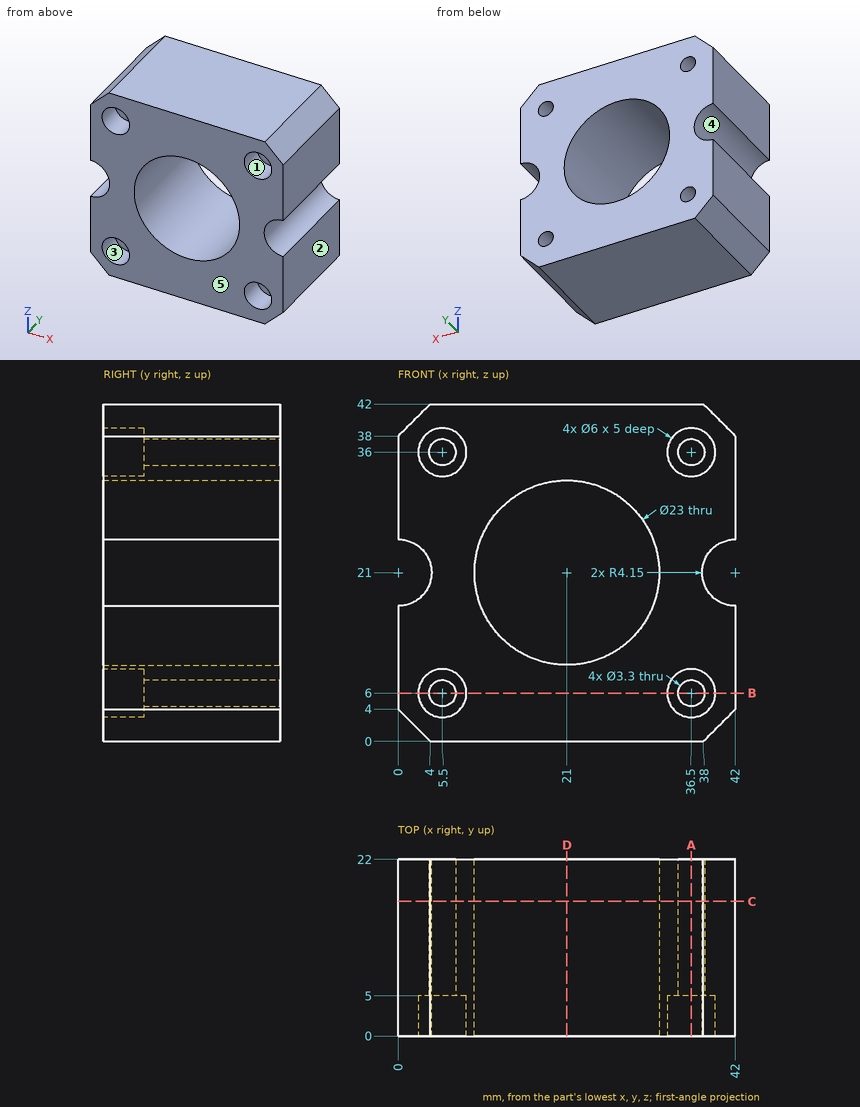
The figure shows three views and two pictorial views of one solid part (mm, origin at its lowest corner). Answer the questions. A direction names the side the tool comes from. Coordinates: 2 decimals unless noted, no trailing zeros. Loops run counter-clockwise (first coordinate to the right, second up) from the corner with the lowest first, then second, coordinate; pieces in that order, holes last. Notation, with made-up numbers: (56, 49.25) -> (109, 49.25) arc R11 cw to (109, 56.25) -> close; hole circle Ø11 at (41.25, 25.25). An arc over 180 degrees is marked (long way). Use one line per item in the form item = value. Start each with the question number.
Item 1: The part is cut by section B-B on z = 6. Determine the outline of the cut face in (x, y).
Item 2: A flat-ended cylindrical pin translates along its axis: pin 1 Ø5.5 at (x, z) = (5.5, 36) entering from -Y. Find the tip coordinate at first contact, or state that the pin passes through.
Item 3: The part is cut by section A-A on x = 36.5. Determine the outline of the cut face in (y, z), then the cut area to 3 significant figures.
Item 4: The mould has two halves that part along X. Classify the marked faces 3, 4 and 5: released by +X, released by -X, zero draft, split by the parting line, or undercut.
Item 5: The part is cut by section C-C on y = 16.75. Determine the outline of the cut face in (x, z), then the cut area to 3 significant figures.
Item 6: A tool of negligible diameter and unlimited length cuts with its end or side. For the marked faces 1 and 2, from which of +Z, -Z, +X, -X, +Y, -Y can it reach the whole face along a straight path? Write none if from no direction.
Item 7: The part is cut by section D-D on x = 21. Determine the outline of the cut face in (y, z), then the cut area to 3 significant figures.
Item 8: Consider L1, parallel to Z at x = 36.5, y = 2.45; L2, parallel to Z at x = 36.5, y = 18.5; L3, parallel to X at y = 15, z = 36. Determine where each line is inside the solid, lowest interval first. Write a range as [from, to].
Answer key:
q1.outline = (0, 0) -> (2.5, 0) -> (2.5, 5) -> (3.85, 5) -> (3.85, 22) -> (0, 22) -> close; (7.15, 5) -> (8.5, 5) -> (8.5, 0) -> (33.5, 0) -> (33.5, 5) -> (34.85, 5) -> (34.85, 22) -> (7.15, 22) -> close; (38.15, 5) -> (39.5, 5) -> (39.5, 0) -> (42, 0) -> (42, 22) -> (38.15, 22) -> close
q2.pin_1 = 5
q3.outline = (0, 0) -> (22, 0) -> (22, 4.35) -> (5, 4.35) -> (5, 3) -> (0, 3) -> close; (0, 9) -> (5, 9) -> (5, 7.65) -> (22, 7.65) -> (22, 34.35) -> (5, 34.35) -> (5, 33) -> (0, 33) -> close; (0, 39) -> (5, 39) -> (5, 37.65) -> (22, 37.65) -> (22, 42) -> (0, 42) -> close
q3.area = 752 mm2
q4.face_3 = undercut
q4.face_4 = released by -X
q4.face_5 = zero draft
q5.outline = (0, 4) -> (4, 0) -> (38, 0) -> (42, 4) -> (42, 16.85) arc R4.15 cw to (42, 25.15) -> (42, 38) -> (38, 42) -> (4, 42) -> (0, 38) -> (0, 25.15) arc R4.15 cw to (0, 16.85) -> close; hole circle Ø3.3 at (5.5, 6); hole circle Ø3.3 at (5.5, 36); hole circle Ø23 at (21, 21); hole circle Ø3.3 at (36.5, 6); hole circle Ø3.3 at (36.5, 36)
q5.area = 1,230 mm2
q6.face_1 = -Y
q6.face_2 = +Z, -Z, +X, +Y, -Y
q7.outline = (0, 0) -> (22, 0) -> (22, 9.5) -> (0, 9.5) -> close; (0, 32.5) -> (22, 32.5) -> (22, 42) -> (0, 42) -> close
q7.area = 418 mm2
q8.L1 = [0, 3], [9, 33], [39, 42]
q8.L2 = [0, 4.35], [7.65, 34.35], [37.65, 42]
q8.L3 = [0, 3.85], [7.15, 34.85], [38.15, 42]
